CAD build for the part. Positions are in the model's coordinates, mm. A direction names the side the tool comes from. Give positions to 0.01 mm unless a question says otherwise; leave off trailing zeros. Write each loop counter-clockwise with the first axis right and the second up, starting at its lowest first coordinate (ties: lowest second). Pieces come first, ordered by that corner, then holes. Notation, with made-up numbers: (-15, -13.5) - (-2, -13.5) arc R20 ccw to (-2, -1.5) - close; hole circle Ø7 at (-29, -2.5). An arc over 180 degrees is marked (long way). Put each result on its own line as item: value. Start each with the question number.
1. Cut at B-B on y = -0.75. List the corners of the cut face in (x, z), and give its area (3 significant figures).
2. Mould opens along X. For faces 5 (the flat face through (0, 1, 8.99)), 6 (the cylindrical face through (-0.14, -5.25, 4.43)), 7 (the cylindrical face through (-3.17, -2.98, 6.33)) say: +X half, -X half, draft (parallel to the pull), parting line (faces both ways), or undercut.
3. Wall check: line 1 (X direction, y = 0, z = 0.65); line 2 (Z direction, x = -2.5, y = -2.75); line 3 (Z direction, x = -2.5, y = 1.75). Give the ranges that are in metal, low to high.
4. Drop flat-ended pins along their axis: pin 1 (1.6 mm diameter, centred on x = 1, y = -0.5, fed in from +Z); pin 2 (1.5 mm diameter, centred on y = -3.5, z = 3.5, fed in from -X); pin 3 (2 mm diameter, centred on x = 2.5, z = 2, fed in from -Y). Give the stop position or say it passes through.
5. Tool access for faces 1 (the flat face through (-0.9, -0.9, 1.24)), 2 (the flat face through (4, 0, 0.5)), 3 (the flat face through (-0.9, 0.7, 1.24)), 4 (the flat face through (0, -1, -0.01)): list every direction of +Z, -Z, +X, -X, +Y, -Y with a clear straight run to the whole face (end or side of a thin tool).
6. Cut at A-A on x = 0. List the corners of the cut face in (y, z), and give its area (3 significant figures).
from build123d import *

# Parameters (mm, degrees)
CYLINDER006_R     = 5.25
CYLINDER006_DEPTH = 9
BOX_W             = 10
BOX_H             = 4
BOX_DEPTH         = 10
CYLINDER007_R     = 3.5
CYLINDER007_DEPTH = 6.5
BOX001_W          = 7.8
BOX001_H          = 1.25
BOX001_DEPTH      = 1.25
CYLINDER008_R     = 0.5
CYLINDER008_DEPTH = 4
CYLINDER009_R     = 0.5
CYLINDER009_DEPTH = 4
CYLINDER012_R     = 0.5
CYLINDER012_DEPTH = 3.5
CYLINDER013_R     = 0.5
CYLINDER013_DEPTH = 4
CYLINDER014_R     = 0.5
CYLINDER014_DEPTH = 4
CYLINDER015_R     = 0.5
CYLINDER015_DEPTH = 3.5
CYLINDER020_R     = 1.5
CYLINDER020_DEPTH = 3
CYLINDER021_R     = 0.45
CYLINDER021_DEPTH = 3
BOX002_W          = 3.2
BOX002_H          = 0.9
BOX002_DEPTH      = 1
CYLINDER022_R     = 0.5
CYLINDER022_DEPTH = 3
BOX003_W          = 1
BOX003_H          = 3
BOX003_DEPTH      = 1
CYLINDER023_R     = 4.35
CYLINDER023_DEPTH = 1


with BuildPart() as part:
    # Cylinder006 → Cylinder006 (join)
    with BuildSketch(Plane.XY.offset(-1.25)):
        Circle(CYLINDER006_R)
    extrude(amount=CYLINDER006_DEPTH)

    # Box → Box (cut)
    with BuildSketch(Plane(origin=(-5, 2, -1.5), x_dir=(1, 0, 0), z_dir=(0, 0, 1))):
        with Locations((5, 2)):
            Rectangle(BOX_W, BOX_H)
    extrude(amount=BOX_DEPTH, mode=Mode.SUBTRACT)

    # Cylinder007 → Cylinder007 (cut)
    with BuildSketch(Plane.XY.offset(1.5)):
        Circle(CYLINDER007_R)
    extrude(amount=CYLINDER007_DEPTH, mode=Mode.SUBTRACT)

    # Box001 → Box001 (join)
    with BuildSketch(Plane(origin=(-3.9, 0.75, 6.5), x_dir=(1, 0, 0), z_dir=(0, 0, 1))):
        with Locations((3.9, 0.625)):
            Rectangle(BOX001_W, BOX001_H)
    extrude(amount=BOX001_DEPTH)

    # Cylinder008 → Cylinder008 (cut)
    with BuildSketch(Plane(origin=(-1, 0, -2), x_dir=(1, 0, 0), z_dir=(0, 0, 1))):
        Circle(CYLINDER008_R)
    extrude(amount=CYLINDER008_DEPTH, mode=Mode.SUBTRACT)

    # Cylinder009 → Cylinder009 (cut)
    with BuildSketch(Plane(origin=(1, 0, -2), x_dir=(1, 0, 0), z_dir=(0, 0, 1))):
        Circle(CYLINDER009_R)
    extrude(amount=CYLINDER009_DEPTH, mode=Mode.SUBTRACT)

    # Cylinder012 → Cylinder012 (cut)
    with BuildSketch(Plane(origin=(-2.4, -1, 5.1), x_dir=(0.382683, -0.92388, 0), z_dir=(-0.92388, -0.382683, 0))):
        Circle(CYLINDER012_R)
    extrude(amount=CYLINDER012_DEPTH, mode=Mode.SUBTRACT)

    # Cylinder013 → Cylinder013 (cut)
    with BuildSketch(Plane(origin=(-0.75, -2, 5.1), x_dir=(0.861629, -0.507538, 0), z_dir=(-0.507538, -0.861629, 0))):
        Circle(CYLINDER013_R)
    extrude(amount=CYLINDER013_DEPTH, mode=Mode.SUBTRACT)

    # Cylinder014 → Cylinder014 (cut)
    with BuildSketch(Plane(origin=(0.75, -2, 5.1), x_dir=(0.861629, 0.507538, 0), z_dir=(0.507538, -0.861629, 0))):
        Circle(CYLINDER014_R)
    extrude(amount=CYLINDER014_DEPTH, mode=Mode.SUBTRACT)

    # Cylinder015 → Cylinder015 (cut)
    with BuildSketch(Plane(origin=(2.4, -1, 5.1), x_dir=(0.382683, 0.92388, 0), z_dir=(0.92388, -0.382683, 0))):
        Circle(CYLINDER015_R)
    extrude(amount=CYLINDER015_DEPTH, mode=Mode.SUBTRACT)

    # Cylinder020 → Cylinder020 (cut)
    with BuildSketch(Plane.XY):
        Circle(CYLINDER020_R)
    extrude(amount=CYLINDER020_DEPTH, mode=Mode.SUBTRACT)

    # Cylinder021 → Cylinder021 (cut)
    with BuildSketch(Plane(origin=(1, 0, -0.75), x_dir=(0, 0, -1), z_dir=(1, 0, 0))):
        Circle(CYLINDER021_R)
    extrude(amount=CYLINDER021_DEPTH, mode=Mode.SUBTRACT)

    # Box002 → Box002 (cut)
    with BuildSketch(Plane(origin=(0.8, -0.45, -1.73), x_dir=(1, 0, 0), z_dir=(0, 0, 1))):
        with Locations((1.6, 0.45)):
            Rectangle(BOX002_W, BOX002_H)
    extrude(amount=BOX002_DEPTH, mode=Mode.SUBTRACT)

    # Cylinder022 → Cylinder022 (join)
    with BuildSketch(Plane(origin=(0, 1.5, 0.45), x_dir=(1, 0, 0), z_dir=(0, -1, 0))):
        Circle(CYLINDER022_R)
    extrude(amount=CYLINDER022_DEPTH)

    # Box003 → Box003 (join)
    with BuildSketch(Plane(origin=(-0.5, -1.5, -0.55), x_dir=(1, 0, 0), z_dir=(0, 0, 1))):
        with Locations((0.5, 1.5)):
            Rectangle(BOX003_W, BOX003_H)
    extrude(amount=BOX003_DEPTH)

    # Cylinder023 → Cylinder023 (cut)
    with BuildSketch(Plane.XY.offset(4.6)):
        Circle(CYLINDER023_R)
    extrude(amount=CYLINDER023_DEPTH, mode=Mode.SUBTRACT)


with BuildPart() as part_1:
    # Body001 placement: moved
    add(part.part.moved(Location((0, 0, 1.24))))


solid = part_1.part
Report:
1. outline: (-5.2, -0.01) - (5.2, -0.01) - (5.2, 8.99) - (3.42, 8.99) - (3.42, 6.84) - (4.28, 6.84) - (4.28, 5.84) - (3.42, 5.84) - (3.42, 2.74) - (1.3, 2.74) - (1.3, 1.24) - (0.5, 1.24) - (0.5, 1.69) arc R0.5 ccw to (-0.5, 1.69) - (-0.5, 1.24) - (-1.3, 1.24) - (-1.3, 2.74) - (-3.42, 2.74) - (-3.42, 5.84) - (-4.28, 5.84) - (-4.28, 6.84) - (-3.42, 6.84) - (-3.42, 8.99) - (-5.2, 8.99) - close
1. area: 46.0 mm²
2. face 5: draft
2. face 6: parting line
2. face 7: undercut
3. line 1: x = -5.25 to -1.5, -0.5 to 0.5, 4 to 5.25
3. line 2: z = -0.01 to 5.84, 6.84 to 8.99
3. line 3: z = -0.01 to 2.74, 7.74 to 8.99
4. pin 1: stops at z = 2.74
4. pin 2: stops at x = -4.47
4. pin 3: stops at y = -5.03
5. face 1: +Z
5. face 2: -Z
5. face 3: none
5. face 4: -Z, +X, -X, +Y, -Y
6. outline: (-5.25, -0.01) - (2, -0.01) - (2, 2.74) - (1.5, 2.74) - (1.5, 2.19) - (-1.5, 2.19) - (-1.5, 2.74) - (-3.5, 2.74) - (-3.5, 5.84) - (-4.35, 5.84) - (-4.35, 6.84) - (-3.5, 6.84) - (-3.5, 8.99) - (-5.25, 8.99) - close; (0.75, 7.74) - (2, 7.74) - (2, 8.99) - (0.75, 8.99) - close
6. area: 29.9 mm²
